```python
from build123d import *

# Parameters (mm, degrees)
SKETCH1_W               = 75
SKETCH1_H               = 75
BOSS_EXTRUDE1_DEPTH     = 8
FILLET1_R               = 10
SKETCH2_R               = 17.5
BOSS_EXTRUDE2_DEPTH     = 37.5
SKETCH3_R               = 17
BOSS_EXTRUDE3_DEPTH     = 200
SKETCH4_R               = 22
SKETCH4_R_2             = 17
BOSS_EXTRUDE4_DEPTH     = 10
BOSS_EXTRUDE5_DEPTH     = 50
SKETCH6_R               = 17.5
CUT_EXTRUDE1_DEPTH      = 25
SKETCH7_R               = 17.5
BOSS_EXTRUDE6_DEPTH     = 100
CUT_EXTRUDE2_DEPTH      = 235.438691346
CUT_EXTRUDE2_DEPTH_BACK = 235.438691346
SKETCH8_R               = 5.5
CUT_EXTRUDE3_DEPTH      = 258.012159245
CUT_EXTRUDE3_DEPTH_BACK = 258.012159245
SKETCH10_R              = 14
CHAMFER1_SIZE           = 5
CUT_EXTRUDE4_DEPTH      = 12
FILLET3_R               = 3
FILLET2_R               = 3


with BuildPart() as part:
    # Sketch1 → Boss-Extrude1 (new body)
    with BuildSketch(Plane.XY):
        Rectangle(SKETCH1_W, SKETCH1_H)
    extrude(amount=BOSS_EXTRUDE1_DEPTH)

    # Fillet1
    fillet1_edges = [part.edges().sort_by_distance(p)[0] for p in [
        (37.5, -37.5, 4),
        (-37.5, -37.5, 4),
        (-37.5, 37.5, 4),
        (37.5, 37.5, 4),
    ]]
    fillet(fillet1_edges, radius=FILLET1_R)

    # Sketch2 → Boss-Extrude2 (add, symmetric)
    with BuildSketch(Plane(origin=(0, 0, 0), x_dir=(1, 0, 0), z_dir=(0, 1, 0))):
        with BuildLine():
            Line((-27.5, -8), (-27.5, -30))
            ThreePointArc((-27.5, -30), (0, -57.5), (27.5, -30))
            Line((27.5, -30), (27.5, -8))
            Line((27.5, -8), (-27.5, -8))
        make_face()
        with Locations(Location((0, -30, 0), (0, 0, 270))):
            Circle(SKETCH2_R, mode=Mode.SUBTRACT)
    extrude(amount=BOSS_EXTRUDE2_DEPTH, both=True)


with BuildPart() as body_2:
    # Sketch3 → Boss-Extrude3 (new body)
    with BuildSketch(Plane(origin=(0, 37.5, 0), x_dir=(1, 0, 0), z_dir=(0, 1, 0))):
        with Locations(Location((0, -30, 0), (0, 0, 270))):
            Circle(SKETCH3_R)
    extrude(amount=-BOSS_EXTRUDE3_DEPTH)

    # Sketch4 → Boss-Extrude4 (add)
    with BuildSketch(Plane.XZ.offset(37.5)):
        with Locations(Location((0, 30, 0), (0, 0, 270))):
            Circle(SKETCH4_R)
        with Locations(Location((0, 30, 0), (0, 0, 90))):
            Circle(SKETCH4_R_2, mode=Mode.SUBTRACT)
    extrude(amount=BOSS_EXTRUDE4_DEPTH)


with BuildPart() as body_3:
    # Sketch5 → Boss-Extrude5 (new body)
    with BuildSketch(Plane.XZ.offset(162.5)):
        with BuildLine():
            Line((-8, 15), (-8, 5))
            Line((-8, 5), (-12.5, 5))
            Line((-12.5, 5), (-25, 17.5))
            Line((-25, 17.5), (-25, 82))
            Line((-25, 82), (0, 82))
            Line((0, 82), (0, 47))
            ThreePointArc((0, 47), (-16.492422502, 34.123105626), (-8, 15))
        make_face()
    extrude(amount=-BOSS_EXTRUDE5_DEPTH)

    # Mirror1: body 3 across plane


with BuildPart() as body_3_1:
    add(body_3.part)
    add(body_3.part.mirror(Plane(origin=(0, -112.5, 82), x_dir=(0, 0, 1), z_dir=(1, 0, 0))))

    # Sketch6 → Cut-Extrude1 (cut)
    with BuildSketch(Plane.XY.offset(82)):
        with Locations((0, -137.5)):
            Circle(SKETCH6_R)
    extrude(amount=-CUT_EXTRUDE1_DEPTH, mode=Mode.SUBTRACT)


with BuildPart() as body_4:
    # Sketch7 → Boss-Extrude6 (new body)
    with BuildSketch(Plane.XY.offset(57)):
        with Locations((0, -137.5)):
            Circle(SKETCH7_R)
    extrude(amount=BOSS_EXTRUDE6_DEPTH)


with BuildPart() as cut_extrude2_tool:
    # Sketch8 → Cut-Extrude2 (new, two sides: drawn at the far end of the back side and taken through both)
    with BuildSketch(Plane(origin=(25, 0, 0), x_dir=(0, 0, -1), z_dir=(1, 0, 0)).offset(-CUT_EXTRUDE2_DEPTH_BACK)):
        with Locations((-30, -137.5)):
            Circle(SKETCH8_R)
    extrude(amount=CUT_EXTRUDE2_DEPTH + CUT_EXTRUDE2_DEPTH_BACK)


with BuildPart() as body_2_1:
    add(body_2.part)

    # Cut-Extrude2: cut by cut_extrude2_tool
    add(cut_extrude2_tool.part, mode=Mode.SUBTRACT)

    # Sketch10 → Cut-Extrude3 (cut, two sides: drawn at the far end of the back side and taken through both)
    with BuildSketch(Plane.XZ.offset(162.5).offset(-CUT_EXTRUDE3_DEPTH_BACK)):
        with Locations(Location((0, 30, 0), (0, 0, 270))):
            Circle(SKETCH10_R)
    extrude(amount=CUT_EXTRUDE3_DEPTH + CUT_EXTRUDE3_DEPTH_BACK, mode=Mode.SUBTRACT)


with BuildPart() as body_3_2:
    add(body_3_1.part)

    # Cut-Extrude2: cut by cut_extrude2_tool
    add(cut_extrude2_tool.part, mode=Mode.SUBTRACT)

    # Chamfer1
    chamfer1_edges = [body_3_2.edges().sort_by_distance(p)[0] for p in [
        (25, -137.5, 35.5),
    ]]
    chamfer(chamfer1_edges, length=CHAMFER1_SIZE)

    # Sketch11 → Cut-Extrude4 (cut)
    with BuildSketch(Plane.ZY.offset(25)):
        Polygon((39, -142.696152423), (39, -132.303847577), (30, -127.107695155), (21, -132.303847577), (21, -142.696152423), (30, -147.892304845), align=None)
    extrude(amount=-CUT_EXTRUDE4_DEPTH, mode=Mode.SUBTRACT)

    # Fillet3
    fillet3_edges = [body_3_2.edges().sort_by_distance(p)[0] for p in [
        (-8, -137.5, 5),
        (-12.5, -137.5, 5),
        (-25, -137.5, 17.5),
        (8, -137.5, 5),
        (12.5, -137.5, 5),
        (25, -137.5, 17.5),
    ]]
    fillet(fillet3_edges, radius=FILLET3_R)

    # Fillet2
    fillet2_edges = [body_3_2.edges().sort_by_distance(p)[0] for p in [
        (12.40540961, -162.5, 5.228361402),
        (-12.40540961, -162.5, 5.228361402),
        (-11.128679656, -112.5, 5),
        (-8, -112.5, 11.5),
        (18.75, -112.5, 11.25),
        (11.128679656, -112.5, 5),
        (8, -112.5, 11.5),
        (-24.771638598, -112.5, 17.59459039),
        (24.771638598, -112.5, 17.59459039),
        (-8.878679656, -112.5, 5.878679656),
        (8.878679656, -112.5, 5.878679656),
        (12.40540961, -112.5, 5.228361402),
        (-12.40540961, -112.5, 5.228361402),
        (-25, -112.5, 50.371320344),
        (25, -162.5, 50.371320344),
        (25, -112.5, 50.371320344),
        (-25, -162.5, 50.371320344),
        (-18.75, -162.5, 11.25),
        (-18.75, -112.5, 11.25),
        (8, -162.5, 11.5),
        (11.128679656, -162.5, 5),
        (18.75, -162.5, 11.25),
        (-11.128679656, -162.5, 5),
        (-8, -162.5, 11.5),
        (-24.771638598, -162.5, 17.59459039),
        (24.771638598, -162.5, 17.59459039),
        (-8.878679656, -162.5, 5.878679656),
        (8.878679656, -162.5, 5.878679656),
    ]]
    fillet(fillet2_edges, radius=FILLET2_R)


solid = part.part
```
Read the model definition and answer for the solid it produces. Units are mm, in the model's axes. A direction names the side the tool comes from. Give positions to 0.01 mm unless a question says otherwise; leave off trailing zeros. Write each loop counter-clockwise with the first axis right and the second up, starting at its lowest first coordinate (ties: lowest second). Pieces come first, ordered by that corner, then holes. Notation, with made-up numbers: M 13.25,17.5 L 21.25,17.5 A19 cw 21.25,38.5 Z; hole C 87,41.25 d7. An arc over 180 degrees is marked long. Put each result on its own line as item: value. Start each with the question number.
1. The part is cut by section B-B, the plane y = 11. Give the vertices of the cut face in (x, z), and give its area (3 significant figures).
2. Which of the six approach directions +Z, -Z, +X, -X, +Y, -Y give full straight-line access (tool end or side, diameter ignored) to faces 1 (the flat face through (-33, 1, 8)), 2 (the flat face through (37.5, 0, 4)), 3 (the flat face through (32, 1, 8))?
3. The part is cut by section C-C, the plane z = 31.5. Give the vertices of the cut face in (x, y).
4. The part is cut by section A-A, the plane x = 0. Give the vertices of the cut face in (y, z), and give its area (3 significant figures).
5. Each of these flat-tipped pins is pushed along its axis until it touches: pin 1 Ø8 at (x, y) = (19, -27) entering from +Z; pin 2 Ø3 at (x, y) = (32.5, 14) entering from +Z; pin 3 Ø12 at (x, y) = (7.5, -23.5) entering from +Z; pin 4 Ø4 at (x, y) = (-13.5, -18) entering from -Z. Where does it stop, or does it pass through?
6. The part is cut by section D-D, the plane x = -22. Give the vertices of the cut face in (y, z), and give its area (3 significant figures).
7. Consider line 1 along X through (y, z) = (4.5, 30); line 2 along X through (y, z) = (20.5, 27); line 3 along Z through (x, y) = (-13.5, -25). Determine where each line is inside the solid, lowest interval first.
Final values:
1. outline: M -37.5,0 L 37.5,0 L 37.5,8 L 27.5,8 L 27.5,30 A27.5 ccw -27.5,30 L -27.5,8 L -37.5,8 Z; hole C 0,30 d35
1. area: 2,040 mm²
2. face 1: +Z, -X, +Y, -Y
2. face 2: +Z, -Z, +X, +Y, -Y
2. face 3: +Z, +X, +Y, -Y
3. outline: M -27.46,-37.5 L -17.44,-37.5 L -17.44,37.5 L -27.46,37.5 Z; M 17.44,-37.5 L 27.46,-37.5 L 27.46,37.5 L 17.44,37.5 Z
4. outline: M -37.5,0 L 37.5,0 L 37.5,12.5 L -37.5,12.5 Z; M -37.5,47.5 L 37.5,47.5 L 37.5,57.5 L -37.5,57.5 Z
4. area: 1,690 mm²
5. pin 1: stops at z = 53.05
5. pin 2: stops at z = 8
5. pin 3: stops at z = 57.46
5. pin 4: stops at z = 0
6. outline: M -37.5,0 L 37.5,0 L 37.5,46.5 L -37.5,46.5 Z
6. area: 3,490 mm²
7. line 1: x = -27.5 to -17.5, 17.5 to 27.5
7. line 2: x = -27.5 to -17.24, 17.24 to 27.5
7. line 3: z = 0 to 18.86, 41.14 to 53.96
